```python
from build123d import *

# Parameters (mm, degrees)
SKETCH_2_R      = 5
SKETCH_2_R_2    = 3
SKETCH_2_W      = 5
SKETCH_2_H      = 12
EXTRUDE_1_DEPTH = 3


with BuildPart() as part:
    # 草图2 → 凸台-拉伸1 (new body)
    # profile 1 of 3: a face of its own
    with BuildSketch(Plane(origin=(0, 0, 0), x_dir=(1, 0, 0), z_dir=(0, 1, 0))):
        Circle(SKETCH_2_R)
        with Locations(Location((0, 0, 0), (0, 0, 270))):
            Circle(SKETCH_2_R_2, mode=Mode.SUBTRACT)
    # profile 2 of 3: a face of its own
    with BuildSketch(Plane(origin=(0, 0, 0), x_dir=(1, 0, 0), z_dir=(0, 1, 0))):
        with Locations((0, -20.660254038)):
            Circle(SKETCH_2_R)
        with Locations(Location((0, -20.660254038, 0), (0, 0, 270))):
            Circle(SKETCH_2_R_2, mode=Mode.SUBTRACT)
    # profile 3 of 3: a face of its own
    with BuildSketch(Plane(origin=(0, 0, 0), x_dir=(1, 0, 0), z_dir=(0, 1, 0))):
        with Locations((0, -10.330127019)):
            Rectangle(SKETCH_2_W, SKETCH_2_H)
    extrude(amount=EXTRUDE_1_DEPTH)


solid = part.part
```
Input: part model. Units: mm. Frame: model coordinates. A direction names the side the tool comes from. Give positions to 0.01 mm unless a question says otherwise; leave off trailing zeros. Loops run counter-clockwise (first coordinate to the right, second up) from the corner with the lowest first, then second, coordinate; pieces in that order, holes last. Notation, with made-up numbers: M 39.5,17.25 L 62.5,17.25 A19 cw 62.5,50.25 Z; hole C 40,51 d9. An arc over 180 degrees is marked long. Answer as CSV lines item,"result". Start each with the question number.
1. Line query: L1, parallel to Z at x = -1.5, y = 1.8; L2, parallel to X at y = 2.4, z = 7.5; L3, parallel to Z at x = 1, y = 2.6. Output: solid intervals per line, ascending.
2. Section D-D on y = 1.25. Return loops of the section in (x, z), plus the area to 3 significant figures.
3. Section B-B on z = 0. Return loops of the section in (x, y).
4. Pin query (flat end, axial travel): P1, Ø1.5, axis at y = 1.5, z = 10, coming from the -X side. Return the tip coordinate at first contact, or that it passes through.
5. Section C-C on x = 4. Return loops of the section in (y, z).
6. Pull-direction query (X, two-part tool) for faces 1 (the face through (0.132, 1.479, 17.663)), 2 (the face through (0, 3, 10)), 3 (the face through (0, 1, -5)); classes: released by +X, released by -X, zero draft, split by the parting line, or undercut.
7. Section A-A on x = 0. Return loops of the section in (y, z).
8. Reachability of faces 4 (the face through (2.5, 1, 10)), 5 (the face through (0.9, 1.48, 2.86)), 6 (the face through (-2.5, 1, 10)) from +Z, -Z, +X, -X, +Y, -Y: full face, straight path, thin tool, end or side. Return the list, or none.
Computed values:
1,L1,"z = -4.77 to -2.6, 2.6 to 18.06, 23.26 to 25.43"
1,L2,"x = -2.5 to 2.5"
1,L3,"z = -4.9 to -2.83, 2.83 to 17.83, 23.49 to 25.56"
2,outline,"M -2.5,4.33 A5 ccw long 2.5,4.33 L 2.5,16.33 A5 ccw long -2.5,16.33 Z; hole C 0,0 d6; hole C 0,20.66 d6"
2,area,"156 mm²"
3,outline,"M -5,0 L -3,0 L -3,3 L -5,3 Z; M 3,0 L 5,0 L 5,3 L 3,3 Z"
4,P1,"stops at x = -2.5"
5,outline,"M 0,-3 L 3,-3 L 3,3 L 0,3 Z; M 0,17.66 L 3,17.66 L 3,23.66 L 0,23.66 Z"
6,face 1,"undercut"
6,face 2,"zero draft"
6,face 3,"split by the parting line"
7,outline,"M 0,-5 L 3,-5 L 3,-3 L 0,-3 Z; M 0,3 L 3,3 L 3,17.66 L 0,17.66 Z; M 0,23.66 L 3,23.66 L 3,25.66 L 0,25.66 Z"
8,face 4,"+X, +Y, -Y"
8,face 5,"+Y, -Y"
8,face 6,"-X, +Y, -Y"
